Autodesk Fusion 360 part; units mm, degrees
sketch "Sketch2" plane through (0, 0, 0) normal (1, 0, 0) x (0, 0, -1)
  line L0 (0, 0) -> (140, 0)
  line L1 (140, 0) -> (140, 15)
  line L2 (140, 15) -> (0, 15)
  line L3 (0, 15) -> (0, 0)
  line L4 (9, 15) -> (-7, 15)
  line L5 (-7, 15) -> (-7, 455)
  line L6 (-7, 455) -> (9, 455)
  line L7 (9, 455) -> (9, 15)
  dimension "d1" = 16
  dimension "d2" = 15
  dimension "d3" = 140
  dimension "d4" = 7
  dimension "d5" = 455
extrude "Extrude1" add sketch "Sketch2" along normal mid plane 110
sketch "Sketch3" plane through (0, 0, 0) normal (1, 0, 0) x (0, 0, -1)
  line L0 (9, 15) -> (9, 455)
  line L1 (140, 15) -> (9, 15)
  line L2 (9, 442.5) -> (21, 442.5)
  line L3 (21, 442.5) -> (127.5, 27)
  line L4 (127.5, 27) -> (127.5, 15)
  dimension "d12" = 12
  dimension "d13" = 12.5
  dimension "d14" = 12.5
  dimension "d15" = 12
extrude "Extrude2" add sketch "Sketch3" along normal mid plane 31.76
sketch "Sketch4" plane through (0, 0, -9) normal (0, 0, -1) x (-1, 0, 0)
  line L0 (-15.88, 15) -> (-15.88, 442.5)
  line L1 (-15.88, 442.5) -> (15.88, 442.5)
  line L2 (15.88, 442.5) -> (15.88, 15)
  line L3 (15.88, 15) -> (55, 15)
  line L4 (55, 15) -> (55, 455)
  line L5 (55, 455) -> (-55, 455)
  line L6 (-55, 455) -> (-55, 15)
  line L7 (-55, 15) -> (-15.88, 15)
  line L8 (0, 455) -> (0, 0) construction
  circle A0 centre (-30, 445) radius 2.5
  circle A1 centre (-30, 410) radius 2.5
  circle A2 centre (-30, 375) radius 2.5
  circle A3 centre (-30, 340) radius 2.5
  circle A4 centre (-30, 305) radius 2.5
  circle A5 centre (-30, 270) radius 2.5
  circle A6 centre (-30, 235) radius 2.5
  circle A7 centre (-30, 200) radius 2.5
  circle A8 centre (-30, 165) radius 2.5
  circle A9 centre (-30, 130) radius 2.5
  circle A10 centre (30, 410) radius 2.5
  circle A11 centre (30, 375) radius 2.5
  circle A12 centre (30, 340) radius 2.5
  circle A13 centre (30, 305) radius 2.5
  circle A14 centre (30, 270) radius 2.5
  circle A15 centre (30, 235) radius 2.5
  circle A16 centre (30, 200) radius 2.5
  circle A17 centre (30, 165) radius 2.5
  circle A18 centre (30, 130) radius 2.5
  circle A19 centre (30, 445) radius 2.5
  dimension "d18" = 30
  dimension "d19" = 5
  dimension "d20" = 10
  dimension "d23" = 35
  dimension "d24" = 0
extrude "Extrude3" cut sketch "Sketch4" against normal blind 100 contours A0 | A1 | A2 | A3 | A4 | A5 | A6 | A7 | A8 | A9 | A10 | A11 | A12 | A13 | A14 | A15 | A16 | A17 | A18 | A19
sketch "Sketch5" plane through (0, 15, 0) normal (0, 1, 0) x (-1, 0, 0)
  line L0 (-15.88, -127.5) -> (-15.88, -9)
  line L1 (-15.88, -9) -> (-55, -9)
  line L2 (-55, -9) -> (-55, -140)
  line L3 (-55, -140) -> (55, -140)
  line L4 (55, -140) -> (55, -9)
  line L5 (55, -9) -> (15.88, -9)
  line L6 (15.88, -9) -> (15.88, -127.5)
  line L7 (15.88, -127.5) -> (-15.88, -127.5)
  circle A0 centre (37, -125) radius 3.9688
  circle A1 centre (37, -95) radius 3.9688
  circle A2 centre (37, -65) radius 3.9688
  circle A3 centre (37, -35) radius 3.9688
  line L8 (37, -125) -> (37, -35) construction
  line L9 (37, -80) -> (52, -80) construction
  line L10 (52, -80) -> (52, -75.9045) construction
  circle A4 centre (67, -125) radius 3.9688
  circle A5 centre (67, -95) radius 3.9688
  circle A6 centre (67, -65) radius 3.9688
  circle A7 centre (67, -35) radius 3.9688
  line L11 (0, -140) -> (0, 0) construction
  line L12 (-52, -80) -> (-52, -75.9045) construction
  circle A8 centre (-67, -95) radius 3.9688
  line L13 (-37, -80) -> (-52, -80) construction
  circle A9 centre (-67, -125) radius 3.9688
  circle A10 centre (-37, -95) radius 3.9688
  circle A11 centre (-37, -65) radius 3.9688
  circle A12 centre (-67, -65) radius 3.9688
  circle A13 centre (-67, -35) radius 3.9688
  circle A14 centre (-37, -35) radius 3.9688
  line L14 (-37, -125) -> (-37, -35) construction
  circle A15 centre (-37, -125) radius 3.9688
  dimension "d27" = 7.9375
  dimension "d28" = 37
  dimension "d29" = 125
  dimension "d30" = 30
  dimension "d31" = 30
  dimension "d32" = 30
  dimension "d33" = 30
sketch "Sketch6" plane through (0, 0, 7) normal (0, 0, 1) x (1, 0, 0)
  circle A0 centre (30, 235) radius 2.5
  circle A1 centre (-30, 200) radius 2.5
  circle A2 centre (30, 270) radius 2.5
  circle A3 centre (-30, 340) radius 2.5
  circle A4 centre (30, 410) radius 2.5
  circle A5 centre (-30, 445) radius 2.5
  circle A6 centre (30, 375) radius 2.5
  circle A7 centre (-30, 270) radius 2.5
  circle A8 centre (-30, 165) radius 2.5
  circle A9 centre (30, 130) radius 2.5
  circle A10 centre (30, 200) radius 2.5
  circle A11 centre (-30, 235) radius 2.5
  circle A12 centre (30, 305) radius 2.5
  circle A13 centre (-30, 375) radius 2.5
  circle A14 centre (30, 445) radius 2.5
  circle A15 centre (-30, 410) radius 2.5
  circle A16 centre (30, 340) radius 2.5
  circle A17 centre (-30, 305) radius 2.5
  circle A18 centre (30, 165) radius 2.5
  circle A19 centre (-30, 130) radius 2.5
  line L0 (-55, 15) -> (55, 15)
  line L1 (55, 15) -> (55, 455)
  line L2 (55, 455) -> (-55, 455)
  line L3 (-55, 455) -> (-55, 15)
sketch "Sketch7" plane through (0, 0, 0) normal (0, -1, 0) x (1, 0, 0)
  line L0 (-55, -140) -> (55, -140)
  line L1 (55, -140) -> (55, 0)
  line L2 (55, 0) -> (-55, 0)
  line L3 (-55, 0) -> (-55, -140)
  circle A0 centre (-35, -120) radius 5.5
  circle A1 centre (35, -120) radius 5.5
  circle A2 centre (-35, -85) radius 5
  circle A3 centre (35, -85) radius 5
  circle A4 centre (-35, -50) radius 5.5
  circle A5 centre (35, -50) radius 5.5
  dimension "d36" = 20
  dimension "d37" = 20
  dimension "d38" = 11
  dimension "d39" = 35
  dimension "d40" = 10
  dimension "d41" = 70
  dimension "d42" = 20
  dimension "d43" = 35
extrude "Extrude5" cut sketch "Sketch7" against normal blind 35 contours A0 | A1 | A2 | A3 | A4 | A5
sketch "Sketch8" plane through (0, 0, 7) normal (0, 0, 1) x (1, 0, 0)
  circle A0 centre (-35, 400) radius 4
  circle A1 centre (35, 400) radius 4
  line L0 (55, 15) -> (55, 455)
  line L1 (-55, 455) -> (-55, 15)
  circle A2 centre (-35, 435) radius 5.5
  circle A3 centre (35, 435) radius 5.5
  circle A4 centre (-35, 365) radius 5.5
  circle A5 centre (35, 365) radius 5.5
  dimension "d46" = 400
  dimension "d47" = 20
  dimension "d48" = 20
  dimension "d49" = 8
  dimension "d50" = 35
  dimension "d51" = 35
  dimension "d52" = 11
  dimension "d53" = 35
  dimension "d54" = 35
extrude "Extrude6" cut sketch "Sketch8" against normal blind 60
equation "d27 = 5 / 16 * 1 in"
Could you check a few things on this model? Use its own coordinates, in mm. A direction names the side the tool comes from. Round coordinates to 2 decimals unless told otherwise and drop trailing zeros. Loops run counter-clockwise (first coordinate to the right, second up) from the corner with the lowest first, then second, coordinate; pieces in that order, holes last. Notation, with made-up numbers: (55.5, 81.5) - (112.5, 81.5) arc R24 ccw to (112.5, 98.5) - close; hole circle Ø7 at (76.5, -16.75). An arc over 180 degrees is marked (long way). Answer in a Markdown table with one row per item. Add a question column.
(1) I need wall thicknesses on line 1 along X through (y, z) = (200, 1); line 2 along X through (y, z) = (435, 0.5); line 3 along Z through (x, y) = (35, 11.25). Which ranges of each line are inside material? Lowest first, please.
(2) If we mould it in two halves opening along Z, with no side actions, what happens to faces 4 (the face through (33.81, 429.63, -0.89)), 5 (the face through (-1, 232, 7)), 6 (the face through (34.284, 7.395, -44.547))? For each: pulls with the +Z half, pulls with the -Z half, needs draft (parallel to the pull), parting line crosses it, or undercut.
(3) If we section it at B-B (z = -37.5): Please give me the cut outline in (x, y).
(4) If we section it at C-C (y = 73.5): Please give me the cut outline in (x, z).
(5) If we section it at A-A (z = -120): Please give me the cut outline in (x, y), plus the area to 3 significant figures.
(6) For faces 1 (the face through (0, 442.5, -15)), 2 (the face through (-1, 8, 0)), 3 (the face through (15.88, 184, -54)), which set-ups out of +Z, -Z, +X, -X, +Y, -Y let a thin tool reach every point of the face, with its end or its side?
(7) I'm going to push flat-ended pins straight in: pin 1 (4 mm diameter, centred on x = 30, y = 235, fed in from +Z); pin 2 (6.5 mm diameter, centred on x = 30, y = 270, fed in from -Z); pin 3 (8 mm diameter, centred on x = 14.5, y = 101, fed in from -Z); pin 4 (17.5 mm diameter, centred on x = -35, z = -120, fed in from +Y). Where does each tip first touch, or does it pass through?
Model answer:
| question | item | result |
|---|---|---|
| 1 | line 1 | x = -55 to -32.5, -27.5 to 27.5, 32.5 to 55 |
| 1 | line 2 | x = -55 to -40.5, -29.5 to 29.5, 40.5 to 55 |
| 1 | line 3 | z = -140 to -125.5, -114.5 to -90, -80 to -55.5, -44.5 to 0 |
| 2 | face 4 | needs draft |
| 2 | face 5 | pulls with the +Z half |
| 2 | face 6 | undercut |
| 3 | outline | (-55, 0) - (55, 0) - (55, 15) - (15.88, 15) - (15.88, 378.13) - (-15.88, 378.13) - (-15.88, 15) - (-55, 15) - close |
| 4 | outline | (-55, -9) - (-15.88, -9) - (-15.88, -115.58) - (15.88, -115.58) - (15.88, -9) - (55, -9) - (55, 7) - (-55, 7) - close |
| 5 | outline | (-55, 0) - (-40.5, 0) - (-40.5, 15) - (-55, 15) - close; (-29.5, 0) - (29.5, 0) - (29.5, 15) - (15.88, 15) - (15.88, 56.26) - (-15.88, 56.26) - (-15.88, 15) - (-29.5, 15) - close; (40.5, 0) - (55, 0) - (55, 15) - (40.5, 15) - close |
| 5 | area | 2,630 mm² |
| 6 | face 1 | -Z, +X, -X, +Y |
| 6 | face 2 | +Z, +X, -X, -Y |
| 6 | face 3 | -Z, +X, +Y |
| 7 | pin 1 | passes through |
| 7 | pin 2 | stops at z = -9 |
| 7 | pin 3 | stops at z = -109.56 |
| 7 | pin 4 | stops at y = 15 |
